from build123d import *

# Parameters (mm, degrees)
PAD002_DEPTH    = 21
SKETCH005_R     = 3
POCKET002_DEPTH = 24
POCKET003_DEPTH = 26.421739
SKETCH007_R     = 1.75
POCKET004_DEPTH = 2.421739
FILLET001_R     = 1
FILLET002_R     = 1
SKETCH008_W     = 17
SKETCH008_H     = 42
PAD003_DEPTH    = 2
SKETCH013_W     = 2
SKETCH013_H     = 10
PAD006_DEPTH    = 8
POCKET007_DEPTH = 22.46137


with BuildPart() as part:
    # Sketch004 → Pad002 (new body, symmetric)
    with BuildSketch(Plane.YZ):
        Polygon((-13.21037, 0), (13.21037, 0), (13.21037, 10), (3.21037, 10), (-13.21037, 14.399924), align=None)
    extrude(amount=PAD002_DEPTH, both=True)

    # Sketch005 (on Face5 of Pad002) → Pocket002 (cut)
    with BuildSketch(Plane(origin=(0, -13.21037, 0), x_dir=(0, 0, -1), z_dir=(0, -1, 0))):
        with Locations((-5.5, -15.5)):
            Circle(SKETCH005_R)
        with Locations((-5.5, 15.5)):
            Circle(SKETCH005_R)
    extrude(amount=-POCKET002_DEPTH, mode=Mode.SUBTRACT)

    # Sketch006 (on Face2 of Pocket002) → Pocket003 (cut, through all)
    with BuildSketch(Plane(origin=(0, -13.21037, 0), x_dir=(0, 0, -1), z_dir=(0, -1, 0))):
        with BuildLine():
            Line((-2, -11.929286), (-2, 11.929286))
            ThreePointArc((-10.5, 15.50003), (-7.436506, 10.890234), (-2, 11.929286))
            Line((-10.5, 15.50003), (-10.5, 19))
            Line((-10.5, 19), (-14.399924, 19))
            Line((-14.399924, 19), (-14.399924, -19))
            Line((-14.399924, -19), (-10.5, -19))
            Line((-10.5, -19), (-10.5, -15.5))
            ThreePointArc((-2, -11.929286), (-7.436492, -10.890228), (-10.5, -15.5))
        make_face()
    extrude(amount=-POCKET003_DEPTH, mode=Mode.SUBTRACT)

    # Sketch007 (on Face21 of Pocket003) → Pocket004 (cut, through all)
    with BuildSketch(Plane(origin=(0, 10.78963, 0), x_dir=(0, 0, -1), z_dir=(0, -1, 0))):
        with Locations((-5.5, 15.5)):
            Circle(SKETCH007_R)
        with Locations((-5.5, -15.5)):
            Circle(SKETCH007_R)
    extrude(amount=-POCKET004_DEPTH, mode=Mode.SUBTRACT)

    # Fillet001
    fillet001_edges = [part.edges().sort_by_distance(p)[0] for p in [
        (-11.929286, 0, 2),
        (11.929286, 0, 2),
    ]]
    fillet(fillet001_edges, radius=FILLET001_R)

    # Fillet002
    fillet002_edges = [part.edges().sort_by_distance(p)[0] for p in [
        (-19, -5.933013, 10.5),
        (19, -5.933013, 10.5),
    ]]
    fillet(fillet002_edges, radius=FILLET002_R)

    # Sketch008 (on Face15 of Fillet002) → Pad003 (join)
    with BuildSketch(Plane(origin=(0, 2.715054, 10.132719), x_dir=(0, -0.965926, 0.258819), z_dir=(0, 0.258819, 0.965926))):
        with Locations((7.987212, 0)):
            Rectangle(SKETCH008_W, SKETCH008_H)
    extrude(amount=PAD003_DEPTH)

    # Sketch013 (on Face10 of Pad003) → Pad006 (join)
    with BuildSketch(Plane.YZ.offset(21)):
        with Locations((-8.25, 5)):
            Rectangle(SKETCH013_W, SKETCH013_H)
        with Locations((-1, 5)):
            Rectangle(SKETCH013_W, SKETCH013_H)
    extrude(amount=PAD006_DEPTH)

    # Sketch014 (on Face33 of Pad006) → Pocket007 (cut, through all)
    with BuildSketch(Plane(origin=(0, -9.25, 0), x_dir=(0, 0, -1), z_dir=(0, -1, 0))):
        with BuildLine():
            ThreePointArc((-2.75, 23.25), (-1, 25), (-2.75, 26.75))
            Line((-2.75, 26.75), (-7.25, 26.75))
            ThreePointArc((-7.25, 26.75), (-9, 25), (-7.25, 23.25))
            Line((-2.75, 23.25), (-7.25, 23.25))
        make_face()
    extrude(amount=-POCKET007_DEPTH, mode=Mode.SUBTRACT)


solid = part.part
CAD build for the part. Positions are in the model's coordinates, mm. A direction names the side the tool comes from. Coordinates: 2 decimals unless noted, no trailing zeros. Order: outer loops, then holes, each group sorted by start corner. A loop starts at its lowest first (then second) coordinate and runs counter-clockwise, first axis right, second up. Notation, with made-up numbers: (71.25, 38.5) -> (105.25, 38.5) arc R33 ccw to (105.25, 68.5) -> close; hole circle Ø11 at (68.5, -0.5). An arc over 180 degrees is marked (long way). Answer in a Markdown table with one row per item.
1) Band-saw the part on D-D (x = 16.5). List the corners of the cut face in (y, z), and give its area (3 significant figures).
Check values:
| item | result |
|---|---|
| outline | (-13.21, 0) -> (13.21, 0) -> (13.21, 4.06) -> (10.79, 4.06) -> (10.79, 2.67) -> (-13.21, 2.67) -> close; (-13.21, 8.33) -> (10.79, 8.33) -> (10.79, 6.94) -> (13.21, 6.94) -> (13.21, 10) -> (3.21, 10) -> (3.73, 11.93) -> (-12.69, 16.33) -> (-13.21, 14.4) -> (1.34, 10.5) -> (-13.21, 10.5) -> close |
| area | 163 mm2 |
2) Mould opens along Z. For faces 1 (the face through (17.235, 11.983, 5.728)), 2 (the face through (0, -13.21, 1)), 3 (the face through (-0.294, -12.955, 15.352)), 4 (the face through (25, -1, 9)) say: pulls with the +Z half, pulls with the -Z half, needs draft (parallel to the pull), parting line crosses it, or undercut.
Check values:
| item | result |
|---|---|
| face 1 | undercut |
| face 2 | needs draft |
| face 3 | pulls with the +Z half |
| face 4 | undercut |
3) Which spindle directions (+Z, -Z, +X, -X, +Y, -Y) get a long thin tool onto all of the face, cutting with end or side? Do faces 5 (the face through (19, -9, 13)), 6 (the face through (23, -7.25, 5)), 7 (the face through (25, -1, 10)), 8 (the face through (25, -1, 1)). Say none if no direction does.
Check values:
| item | result |
|---|---|
| face 5 | -Y |
| face 6 | +Z, -Z, +X |
| face 7 | +Z, +X, +Y, -Y |
| face 8 | +Y, -Y |
4) Flat gauge pins, fed straight in: P1, Ø0.6, axis at x = 26.5, y = -1, coming from the +Z side; P2, Ø2.5, axis at x = 26.5, z = 7, coming from the -Y side; P3, Ø3, axis at y = -10, z = 13.5, coming from the +X side. Where does each tip first touch, or does it go through?
Check values:
| item | result |
|---|---|
| P1 | z = 10 |
| P2 | y = -9.25 |
| P3 | x = 21 |
5) Band-saw the part on A-A (x = 6). List the corners of the cut face in (y, z), and give its area (3 significant figures).
Check values:
| item | result |
|---|---|
| outline | (-13.21, 0) -> (13.21, 0) -> (13.21, 2) -> (-13.21, 2) -> close; (-13.21, 14.4) -> (3.21, 10) -> (3.73, 11.93) -> (-12.69, 16.33) -> close |
| area | 86.8 mm2 |
6) Band-saw the part on C-C (z = 5.5). Give the number of separate pieces and of enclosed holes in the cut face, and give its area (3 significant figures).
Check values:
| item | result |
|---|---|
| separate pieces | 6 |
| enclosed holes | 0 |
| area | 268 mm2 |
7) Drill centre lines: line 1 (X direction, y = 12.35, z = 5.5); line 2 (Z direction, x = -15, y = -4.25); line 3 (X direction, y = 11.5, z = 4.5). Where is each one in solid material? Low to high.
Check values:
| item | result |
|---|---|
| line 1 | -21 to -17.25, -13.75 to -10.5, 10.5 to 13.75, 17.25 to 21 |
| line 2 | 0 to 2.54, 8.46 to 10.47, 12 to 14.07 |
| line 3 | -21 to -16.94, -14.06 to -10.6, 10.6 to 14.06, 16.94 to 21 |
8) Band-saw the part on B-B (y = 0.75). List the corners of the cut face in (x, z).
Check values:
| item | result |
|---|---|
| outline | (-21, 0) -> (21, 0) -> (21, 12.73) -> (-21, 12.73) -> close; hole (-18.54, 10.66) arc R1 ccw to (-18, 10.5) -> (-15.5, 10.5) arc R5 cw to (-10.95, 3.42) arc R1 ccw to (-10.05, 2) -> (10.05, 2) arc R1 ccw to (10.95, 3.42) arc R5 cw to (15.5, 10.5) -> (18, 10.5) arc R1 ccw to (18.54, 10.66) -> close; hole circle Ø6 at (-15.5, 5.5); hole circle Ø6 at (15.5, 5.5) |
